Read the model definition and answer for the solid it produces. Units are mm, in the model's axes. A direction names the side the tool comes from. Give positions to 0.01 mm unless a question says otherwise; leave off trailing zeros. Write each loop counter-clockwise with the first axis right and the second up, starting at its lowest first coordinate (ties: lowest second). Pieces come first, ordered by that corner, then holes. Notation, with made-up numbers: (63.25, 53) -> (82.25, 53) arc R23 ccw to (82.25, 76) -> close; hole circle Ø3 at (11, 31). An arc over 180 degrees is marked (long way). Use a Markdown table: item, result.
from build123d import *

# Parameters (mm, degrees)
BOSS_EXTRUDE1_DEPTH = 4
FILLET5_R           = 2
SKETCH3_R           = 4
BOSS_EXTRUDE2_DEPTH = 4
CUT_EXTRUDE1_START  = -8
CUT_EXTRUDE1_DEPTH  = 8
CUT_EXTRUDE2_REACH  = 74.805


with BuildPart() as part:
    # Sketch2 → Boss-Extrude1 (new body)
    with BuildSketch(Plane(origin=(0, 0, 0), x_dir=(1, 0, 0), z_dir=(0, 1, 0))):
        with BuildLine():
            Line((-19.444698737, 54.4597806), (-19.444698737, 28.4597806))
            Line((-19.444698737, 28.4597806), (5.602062826, -61.368686618))
            ThreePointArc((5.602062826, -61.368686618), (8.649467973, -65.855333302), (13.789742047, -67.585726043))
            Line((13.789742047, -67.585726043), (17.359306877, -67.585726043))
            ThreePointArc((17.359306877, -67.585726043), (23.466476793, -64.997787917), (25.854828389, -58.809837951))
            Line((25.854828389, -58.809837951), (22.177110502, 54.439455621))
            Line((22.177110502, 54.439455621), (22.802984938, 54.4597806))
            Line((22.802984938, 54.4597806), (-19.444698737, 54.4597806))
        make_face()
    extrude(amount=BOSS_EXTRUDE1_DEPTH)

    # Fillet5
    fillet5_edges = [part.edges().sort_by_distance(p)[0] for p in [
        (24.015969445, 4, 2.185191165),
        (23.466476793, 4, 64.997787917),
        (15.574524462, 4, 67.585726043),
        (8.649467973, 4, 65.855333302),
        (24.015969445, 0, 2.185191165),
        (23.466476793, 0, 64.997787917),
        (15.574524462, 0, 67.585726043),
        (8.649467973, 0, 65.855333302),
        (-19.444698737, 2, -28.4597806),
        (-6.921317955, 4, 16.454453009),
        (-6.921317955, 0, 16.454453009),
    ]]
    fillet(fillet5_edges, radius=FILLET5_R - 0.0001)  # a hair under: the kernel refuses the full size

    # Sketch3 → Boss-Extrude2 (add)
    with BuildSketch(Plane.XZ):
        with Locations(Location((-9.881069751, -35.033682073, 0), (0, 0, 90))):
            Circle(SKETCH3_R)
    extrude(amount=BOSS_EXTRUDE2_DEPTH)

    # Sketch4 → Cut-Extrude1 (cut)
    with BuildSketch(Plane(origin=(0, 4, 0), x_dir=(1, 0, 0), z_dir=(0, 1, 0)).offset(CUT_EXTRUDE1_START)):
        Polygon((23.237390651, 21.78986649), (-2.479011749, 54.4597806), (-19.444698737, 41.566075464), (-32.323067486, 58.511582656), (23.237390651, 102.246472628), (62.340489493, 52.570205291), align=None)
    extrude(amount=CUT_EXTRUDE1_DEPTH, mode=Mode.SUBTRACT)

    # Sketch5 → Cut-Extrude2 (cut, up to next)
    with BuildSketch(Plane(origin=(0, 4, 0), x_dir=(1, 0, 0), z_dir=(0, 1, 0)), mode=Mode.PRIVATE) as cut_extrude2_sk1:
        Polygon((10.216290077, 38.331769621), (-12.707477704, 46.686277287), (-5.274739107, 62.107031808), align=None)
    cut_extrude2_tool1 = extrude(cut_extrude2_sk1.sketch, amount=-CUT_EXTRUDE2_REACH, mode=Mode.PRIVATE) & part.part
    # Sketch5 → Cut-Extrude2 (cut, up to next)
    with BuildSketch(Plane(origin=(0, 4, 0), x_dir=(1, 0, 0), z_dir=(0, 1, 0)), mode=Mode.PRIVATE) as cut_extrude2_sk2:
        Polygon((-19.444698737, 33.221694621), (-7.48638486, 25.86937143), (-13.167620162, 23.386461187), (-19.9430193, 23.807293431), align=None)
    cut_extrude2_tool2 = extrude(cut_extrude2_sk2.sketch, amount=-CUT_EXTRUDE2_REACH, mode=Mode.PRIVATE) & part.part
    add(cut_extrude2_tool1.solids().sort_by_distance((-2.588642, 4, -49.041693))[0], mode=Mode.SUBTRACT)
    add(cut_extrude2_tool2.solids().sort_by_distance((-15.327917, 4, -27.167771))[0], mode=Mode.SUBTRACT)


solid = part.part
Item 1: For a pull along Z with two mould halves and no side action, classify faces 1 (the face through (7, 0, 9)), 2 (the face through (-15.61, 2.03, -23.54)), 3 (the face through (15.6, 0.601, 67.015)) as +Z half, -Z half, draft (parallel to the pull), parting line (faces both ways), or undercut.
Return value:
| item | result |
|---|---|
| face 1 | draft |
| face 2 | undercut |
| face 3 | +Z half |
Item 2: A tool of negligible diameter and unlimited length cuts with its end or side. For faces 4 (the face through (-8.35, -1.97, -31.34)), 5 (the face through (-10, -4, -35)), 6 (the face through (-13.549, 2.028, -29.597)), 7 (the face through (23.91, 0.6, 16.59)), 8 (the face through (23.91, 3.4, 16.59)), from which of +Z, -Z, +X, -X, +Y, -Y can it reach the whole face along a straight path? Write none if from no direction.
Return value:
| item | result |
|---|---|
| face 4 | -Y |
| face 5 | +Z, -Z, +X, -X, -Y |
| face 6 | -X, +Y, -Y |
| face 7 | -Z, +X, -Y |
| face 8 | -Z, +X, +Y |
Item 3: Each of these flat-tipped pins is pushed along its axis until it touches: P1, Ø3, axis at x = 20, y = -0.5, coming from the +Z side; P2, Ø8, axis at x = 21, z = -23.5, coming from the -Y side; P3, Ø1.5, axis at x = -7, z = 13.5, coming from the +Y side. Where does it stop, or does it pass through?
Return value:
| item | result |
|---|---|
| P1 | z = 66.98 |
| P2 | y = 0 |
| P3 | y = 3.93 |
Item 4: A cutting plane is placed at C-C (z = -30). Give the vertices of the cut face in (x, y).
Return value:
| item | result |
|---|---|
| outline | (-14.2, 0) -> (16.77, 0) -> (16.77, 4) -> (-14.2, 4) -> close |
Item 5: A cutting plane is placed at B-B (y = -3). Give the vertices of the cut face in (x, z).
Return value:
| item | result |
|---|---|
| outline | circle Ø8 at (-9.88, -35.03) |
Item 6: Straight lines are drawn through the part: line 1 along Y through (x, z) = (-8.5, -5.5); line 2 along X through (y, z) = (3, -17.5); line 3 along Z through (x, y) = (18, 2.75). For each, find the intervals that lie inside material, in ascending order. Write a range as [from, to].
Return value:
| item | result |
|---|---|
| line 1 | [0, 4] |
| line 2 | [-16.11, 23.11] |
| line 3 | [-28.44, 67.42] |
